Geometry: final body of the model. Coordinates: model frame, mm. A direction names the side the tool comes from. Round coordinates to 2 decimals unless told otherwise and drop trailing zeros. Write each loop counter-clockwise with the first axis right and the second up, starting at its lowest first coordinate (ties: lowest second). Pieces come first, ordered by that corner, then holes. Notation, with made-up numbers: M 68,-24.5 L 75,-24.5 A30 ccw 75,14.5 Z; hole C 61.25,26.25 d5. An arc over 180 degrees is marked long. Answer as CSV lines item,"result". Start each with the question number.
Q1. Section query C-C on z = -7.5. Output: boundary loops of the cut face in (x, y) (3 decimals).
Q2. First-contact query: pin 1 (1 mm diameter, centred on y = -29.5, z = 5, fed in from +X) (3 decimals); pin 2 (1.8 mm diameter, centred on x = -6, y = -20, fed in from +Z); pin 3 (5 mm diameter, centred on x = -1.5, y = -12.5, fed in from +Z). Flat tips, straight axial feed; report the tip coordinate or a pass-through.
Q3. Section query D-D on y = -4. Output: boundary loops of the cut face in (x, z) (3 decimals).
Q4. Section query B-B on x = -3.5. Output: boundary loops of the cut face in (y, z) (3 decimals), and give its area (3 significant figures).
Q5. Reachability of faces 1 (the flat face through (-7.5, -12, -9)), 2 (the flat face through (-13.028, -29.021, 2.767)), 3 (the flat face through (10.2, -21, 11)) from +Z, -Z, +X, -X, +Y, -Y: full face, straight path, thin tool, end or side. Return the list, or none.
Q6. Mould query, pull axis Z, two halves, no side actions, for faces 4 (the flat face through (-13.028, -16.545, 5.692)), 5 (the flat face through (-15, -17, 7)). Classes: pulls with the +Z half, pulls with the -Z half, needs draft (parallel to the pull), parting line crosses it, or undercut.
Q7. Ray query, probe 1 along Z at (x, y) = (0, -1.65) (3 decimals); probe 2 along X at (y, z) = (-11.5, 10.25); probe 3 along Z at (x, y) = (-4.1, -14) (3 decimals). Return the intervals inside material, ascending.
Q8. Section query A-A on y = -26.5. Output: boundary loops of the cut face in (x, z) (1 decimal), and give its area (3 significant figures).
```python
from build123d import *

# Parameters (mm, degrees)
F0_R     = 2.125
F1_DEPTH = 5
F3_DEPTH = 4
F5_DEPTH = 25
F6_R     = 2.125
F7_DEPTH = 25
F9_DEPTH = 4
F10_SIZE = 10


with BuildPart() as f1:
    # F0 (on Front) → F1 (new body)
    with BuildSketch(Plane.XZ):
        Polygon((-7.5, -12.7), (7.5, -12.7), (7.5, -4.7), (15, 0.7), (15, 12.7), (-15, 12.7), (-15, 0.7), (-7.5, -4.7), align=None)
        with Locations((0, -7.5)):
            Circle(F0_R, mode=Mode.SUBTRACT)
        with Locations((0, 5)):
            Circle(F0_R, mode=Mode.SUBTRACT)
    extrude(amount=F1_DEPTH)

    # F2 (on face) → F3 (join)
    with BuildSketch(Plane.XZ.offset(5)):
        Polygon((15, 12.7), (-15, 12.7), (-15, 0.7), (-7.5, -4.7), (-7.5, -12.7), (7.5, -12.7), (7.5, -4.7), (15, 0.7), align=None)
        Polygon((0, -4.122501), (2.925, -5.81125), (2.925, -9.18875), (0, -10.877499), (-2.925, -9.18875), (-2.925, -5.81125), align=None, mode=Mode.SUBTRACT)
        Polygon((0, 8.377499), (2.925, 6.68875), (2.925, 3.31125), (0, 1.622501), (-2.925, 3.31125), (-2.925, 6.68875), align=None, mode=Mode.SUBTRACT)
    extrude(amount=F3_DEPTH)

    # F4 (on face) → F5 (join)
    with BuildSketch(Plane.XZ.offset(9)):
        Polygon((-7.2, -0.8), (-7.2, 12.7), (-15, 12.7), (-15, 0.7), (-7.5, -4.7), (-7.5, -12.7), (-2.925, -12.7), (-2.925, 3.31125), (-2.925, 6.68875), (-2.925, 8.377499), (10.2, 8.377499), (10.2, 12.7), (6.3, 12.7), (6.3, 10.5), (-5, 10.5), (-5, -0.8), align=None)
    extrude(amount=F5_DEPTH)

    # F6 (on face) → F7 (cut)
    with BuildSketch(Plane.YZ.offset(-2.925)):
        with Locations((-26.5, 4.25)):
            Circle(F6_R)
        with Locations((-14, 4.25)):
            Circle(F6_R)
    extrude(amount=-F7_DEPTH, mode=Mode.SUBTRACT)

    # F8 (on face) → F9 (cut)
    with BuildSketch(Plane(origin=(-15, 0, 0), x_dir=(0, -1, 0), z_dir=(-1, 0, 0))):
        Polygon((15.68875, 7.175), (12.31125, 7.175), (10.622501, 4.25), (12.31125, 1.325), (15.68875, 1.325), (17.377499, 4.25), align=None)
        Polygon((28.18875, 7.175), (24.81125, 7.175), (23.122501, 4.25), (24.81125, 1.325), (28.18875, 1.325), (29.877499, 4.25), align=None)
    extrude(amount=-F9_DEPTH, mode=Mode.SUBTRACT)

    # F10
    f10_edges = [f1.edges().sort_by_distance(p)[0] for p in [
        (-5.2125, -34, -12.7),
    ]]
    chamfer(f10_edges, length=F10_SIZE)


solid = f1.part
```
Entries:
1,outline,"M -7.5,-29.2 L -2.925,-29.2 L -2.925,-5 L -2.125,-5 L -2.125,0 L -7.5,0 Z; M 2.125,-5 L 2.925,-5 L 2.925,-9 L 7.5,-9 L 7.5,0 L 2.125,0 Z"
2,pin 1,"stops at x = -2.925"
2,pin 2,"stops at z = -0.8"
2,pin 3,"stops at z = 10.5"
3,outline,"M -15,0.7 L -7.5,-4.7 L -7.5,-12.7 L 7.5,-12.7 L 7.5,-4.7 L 15,0.7 L 15,12.7 L -15,12.7 Z; hole C 0,-7.5 d4.25; hole C 0,5 d4.25"
4,outline,"M -34,-2.7 L -24,-12.7 L 0,-12.7 L 0,12.7 L -9,12.7 L -9,10.5 L -34,10.5 Z; hole C -26.5,4.25 d4.25; hole C -14,4.25 d4.25"
4,area,"730 mm^2"
5,face 1,"-Z, -X, +Y, -Y"
5,face 2,"-X"
5,face 3,"+Z, -Z, +X, -Y"
6,face 4,"undercut"
6,face 5,"needs draft"
7,probe 1,"z = -12.7 to -9.625, -5.375 to 2.875, 7.125 to 12.7"
7,probe 2,"x = -15 to -7.2, -5 to 10.2"
7,probe 3,"z = -12.7 to 2.125, 6.375 to 10.5"
8,outline,"M -15,0.7 L -7.5,-4.7 L -7.5,-10.2 L -2.9,-10.2 L -2.9,2.1 L -5,2.1 L -5,-0.8 L -7.2,-0.8 L -7.2,2.1 L -11,2.1 L -11,1.3 L -15,1.3 Z; M -15,7.2 L -11,7.2 L -11,6.4 L -7.2,6.4 L -7.2,12.7 L -15,12.7 Z; M -5,6.4 L -2.9,6.4 L -2.9,8.4 L 10.2,8.4 L 10.2,12.7 L 6.3,12.7 L 6.3,10.5 L -5,10.5 Z"
8,area,"169 mm^2"
